```python
from build123d import *

# Parameters (mm, degrees)
F0_R     = 3
F1_DEPTH = 6
F2_SIZE  = 0.5
F4_DEPTH = 4


with BuildPart() as f1:
    # F0 (on Top) → F1 (new body, symmetric)
    with BuildSketch(Plane.XY):
        Circle(F0_R)
    extrude(amount=F1_DEPTH, both=True)

    # F2
    f2_edges = [f1.edges().sort_by_distance(p)[0] for p in [
        (-3, 0, 6),
        (-3, 0, -6),
    ]]
    chamfer(f2_edges, length=F2_SIZE)

    # F3 (on face) → F4 (cut)
    with BuildSketch(Plane(origin=(0, 0, -6), x_dir=(1, 0, 0), z_dir=(0, 0, -1))):
        Polygon((0.866025, 1.5), (-0.866025, 1.5), (-1.732051, 0), (-0.866025, -1.5), (0.866025, -1.5), (1.732051, 0), align=None)
    extrude(amount=-F4_DEPTH, mode=Mode.SUBTRACT)


solid = f1.part
```
Here's how the part is built. I have some questions about the finished solid (model axes, mm). A direction names the side the tool comes from. Coordinates: 2 decimals unless noted, no trailing zeros. Order: outer loops, then holes, each group sorted by start corner. A loop starts at its lowest first (then second) coordinate and runs counter-clockwise, first axis right, second up. Notation, with made-up numbers: (8, 20) - (56, 20) arc R21 cw to (56, 27) - close; hole circle Ø5 at (80, 45.25). An arc over 180 degrees is marked (long way). One line per question, with ' | ' between items. Start each with the question number.
1. Please list where these lines run through material, in increasing order: line 1 along Y through (x, z) = (-0.15, -4.5); line 2 along Y through (x, z) = (1, -3); line 3 along Z through (x, y) = (-0.8, 0.65). Write a range as [from, to].
2. Which directions (+Z, -Z, +X, -X, +Y, -Y) give clear straight access to the entire face, cutting with the end or side of a thin tool? Please do faces 1 (the flat face through (0, 0, 6)), 2 (the flat face through (-1.293, -0.76, -4.028)).
3. If we section it at C-C (z = 4.75): Write out the boundary of the cut face in (x, y), and give its area (3 significant figures).
4. If we mould it in two halves opening along X, with no side actions, what happens to faces 3 (the cylindrical face through (-3, 0, 0)), 4 (the flat face through (0, -1.5, -4)), 5 (the flat face through (-1.305, 0.74, -4.028)), 6 (the flat face through (0, -2, -6))? For each: released by +X, released by -X, zero draft, split by the parting line, or undercut.
5. If we section it at B-B (x = 0): Write out the boundary of the cut face in (y, z), and give its area (3 significant figures).
6. I'm going to push flat-ended pins straight in: pin 1 Ø2 at (x, z) = (-1.5, -1.5) entering from -Y; pin 2 Ø1.5 at (x, y) = (0.5, 0.5) entering from -Z. Where does each tip first touch, or does it pass through?
7. If we section it at A-A (z = -4.75): Write out the boundary of the cut face in (x, y).
Model answer:
1) line 1: y = [-3, -1.5], [1.5, 3] | line 2: y = [-2.83, -1.27], [1.27, 2.83] | line 3: z = [-2, 6]
2) face 1: +Z, +X, -X, +Y, -Y | face 2: -Z
3) outline: circle Ø6 at (0, 0) | area: 28.3 mm²
4) face 3: split by the parting line | face 4: undercut | face 5: undercut | face 6: zero draft
5) outline: (-3, -5.5) - (-2.5, -6) - (-1.5, -6) - (-1.5, -2) - (1.5, -2) - (1.5, -6) - (2.5, -6) - (3, -5.5) - (3, 5.5) - (2.5, 6) - (-2.5, 6) - (-3, 5.5) - close | area: 59.5 mm²
6) pin 1: stops at y = -2.96 | pin 2: stops at z = -2
7) outline: circle Ø6 at (0, 0); hole (-1.73, 0) - (-0.87, -1.5) - (0.87, -1.5) - (1.73, 0) - (0.87, 1.5) - (-0.87, 1.5) - close
